Geometry: see drawing. Coordinates: mm, zero at the bounding-box minimum. A direction names the side the tool comes from. Give positions to 0.01 mm unless a question says otherwise; leave off trailing zeros. Write each loop counter-clockwise with the first axis right and the second up, starting at its lowest first coordinate (ties: lowest second). Pieces come first, ordered by that corner, then holes. Notation, with made-up numbers: (-31, 72.5) -> (-11, 72.5) arc R14 cw to (-11, 82.5) -> close; hole circle Ø11 at (19, 45.5). An arc over 180 degrees is marked (long way). Use CSV: the item, a comma, the result in double quotes. Start each with the question number.
1) Section A-A (x = 6). Output: boundary loops of the cut face in (y, z), plus the area to 3 significant figures.
2) Section C-C (y = 9.25). Output: boundary loops of the cut face in (x, z), plus the area to 3 significant figures.
3) Set-up query: the marked faces 1 and 2. Return all of +Z, -Z, +X, -X, +Y, -Y with unobstructed straight access to the full face (end or side cutting, diameter ignored); none if empty.
4) Material intervals for line 1 (X direction, y = 1.25, z = 5.25); line 2 (Y direction, x = 44, z = 11); line 3 (Z direction, x = 24, y = 17), sorted ascending. Write a range as [from, to].
5) Contact query for flat-ended pins moving along their axis: P1, Ø4, axis at x = 44, y = 16, coming from the -Z side; P2, Ø6, axis at x = 47.5, z = 6, coming from the +Y side; P3, Ø2, axis at x = 34, z = 3, coming from the +Y side. Output: stop coordinate, or through.
6) Section B-B (z = 8). Output: boundary loops of the cut face in (x, y).
7) Section D-D (y = 13.25). Output: boundary loops of the cut face in (x, z), plus the area to 3 significant figures.
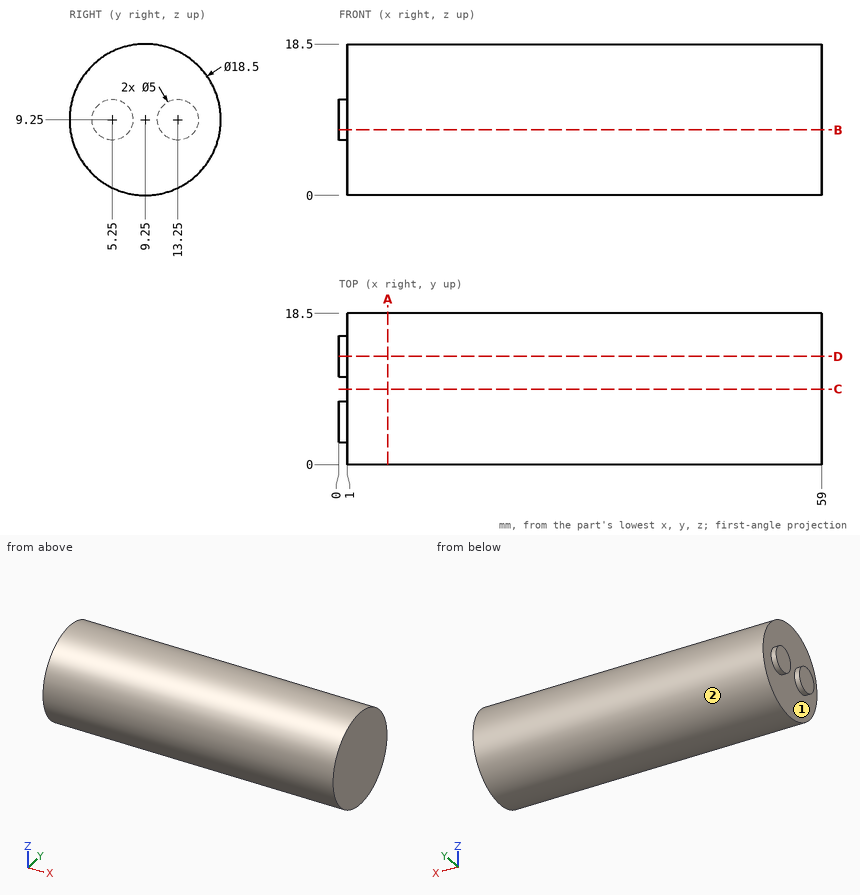
Answers follow:
1,outline,"circle Ø18.5 at (9.25, 9.25)"
1,area,"269 mm^2"
2,outline,"(1, 0) -> (59, 0) -> (59, 18.5) -> (1, 18.5) -> close"
2,area,"1,070 mm^2"
3,face 1,"-X"
3,face 2,"+X, -X"
4,line 1,"x = [1, 59]"
4,line 2,"y = [0.17, 18.33]"
4,line 3,"z = [4.2, 14.3]"
5,P1,"stops at z = 1.31"
5,P2,"stops at y = 18.5"
5,P3,"stops at y = 16.87"
6,outline,"(0, 3.08) -> (1, 3.08) -> (1, 0.08) -> (59, 0.08) -> (59, 18.42) -> (1, 18.42) -> (1, 15.42) -> (0, 15.42) -> (0, 11.08) -> (1, 11.08) -> (1, 7.42) -> (0, 7.42) -> close"
7,outline,"(0, 6.75) -> (1, 6.75) -> (1, 0.91) -> (59, 0.91) -> (59, 17.59) -> (1, 17.59) -> (1, 11.75) -> (0, 11.75) -> close"
7,area,"972 mm^2"
